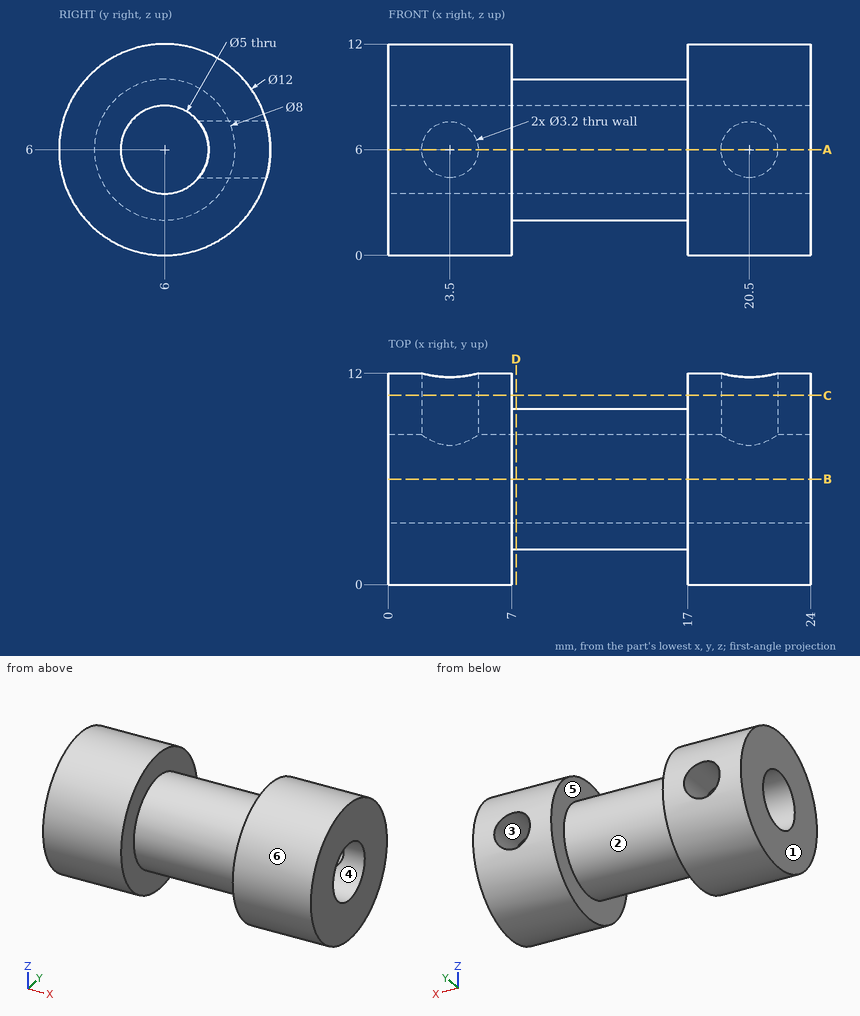
Answer from the drawing. Dimensions are ordinates in mm from the lowest x, y and z of the part. A direction names the side the tool comes from. Give positions to 0.01 mm unless a question says otherwise; leave off trailing zeros. Loops run counter-clockwise (first coordinate to the right, second up) from the corner with the lowest first, then second, coordinate; pieces in that order, holes last. Notation, with made-up numbers: (35.5, 36) - (82.5, 36) arc R22 cw to (82.5, 64) - close; hole circle Ø8 at (65.25, 51.5). An arc over 180 degrees is marked (long way). Answer as CSV lines item,"result". Start each with the question number.
Item 1: A cutting plane is placed at C-C on y = 10.75. Determine the outline of the cut face in (x, z).
Item 2: A cutting plane is placed at B-B on y = 6. Determine the outline of the cut face in (x, z), then the cut area to 3 significant figures.
Item 3: The mould has two halves that part along Z. Classify the marked faces 4, 5 and 6: +Z half, -Z half, draft (parallel to the pull), parting line (faces both ways), or undercut.
Item 4: Each of these flat-tipped pins is pushed along its axis until it touches: pin 1 (2 mm diameter, centred on x = 11.5, y = 6.5, fed in from -Z); pin 2 (5 mm diameter, centred on x = 15, z = 5.5, fed in from +Y); pin 3 (3 mm diameter, centred on y = 6, z = 6, fed in from +X); pin 4 (3 mm diameter, centred on x = 3.5, z = 6, fed in from +Y). Where does it stop, or does it pass through?
Item 5: Find the intervals of material crossed by line 1 (X direction, y = 11.05, z = 6); line 2 (Y direction, x = 9.25, z = 6); line 3 (X direction, y = 9.6, z = 6), in increasing order. Write a range as from..to.
Item 6: For the marked faces 1, 2 and 3, determine the directions among +Z, -Z, +X, -X, +Y, -Y from which every point of the face is accessible in a straight line to the end or side of a thin tool.
Item 7: A cutting plane is placed at A-A on z = 6. Determine the outline of the cut face in (x, y), then the cut area to 3 significant figures.
Item 8: A cutting plane is placed at D-D on x = 7.25. Determine the outline of the cut face in (y, z), then the cut area to 3 significant figures.
Found:
1,outline,"(0, 2.33) - (7, 2.33) - (7, 9.67) - (0, 9.67) - close; (17, 2.33) - (24, 2.33) - (24, 9.67) - (17, 9.67) - close; hole circle Ø3.2 at (3.5, 6); hole circle Ø3.2 at (20.5, 6)"
2,outline,"(0, 0) - (7, 0) - (7, 2) - (17, 2) - (17, 0) - (24, 0) - (24, 3.5) - (0, 3.5) - close; (0, 8.5) - (24, 8.5) - (24, 12) - (17, 12) - (17, 10) - (7, 10) - (7, 12) - (0, 12) - close"
2,area,"128 mm^2"
3,face 4,"undercut"
3,face 5,"draft"
3,face 6,"parting line"
4,pin 1,"stops at z = 2"
4,pin 2,"stops at y = 12"
4,pin 3,"passes through"
4,pin 4,"stops at y = 4"
5,line 1,"x = 0..1.9, 5.1..7, 17..18.9, 22.1..24"
5,line 2,"y = 2..3.5, 8.5..10"
5,line 3,"x = 0..1.9, 5.1..18.9, 22.1..24"
6,face 1,"+Z, -Z, -X, +Y, -Y"
6,face 2,"none"
6,face 3,"+Y"
7,outline,"(0, 0) - (7, 0) - (7, 2) - (17, 2) - (17, 0) - (24, 0) - (24, 3.5) - (0, 3.5) - close; (0, 8.5) - (1.9, 8.5) - (1.9, 12) - (0, 12) - close; (5.1, 8.5) - (18.9, 8.5) - (18.9, 12) - (17, 12) - (17, 10) - (7, 10) - (7, 12) - (5.1, 12) - close; (22.1, 8.5) - (24, 8.5) - (24, 12) - (22.1, 12) - close"
7,area,"106 mm^2"
8,outline,"circle Ø8 at (6, 6); hole circle Ø5 at (6, 6)"
8,area,"30.6 mm^2"
